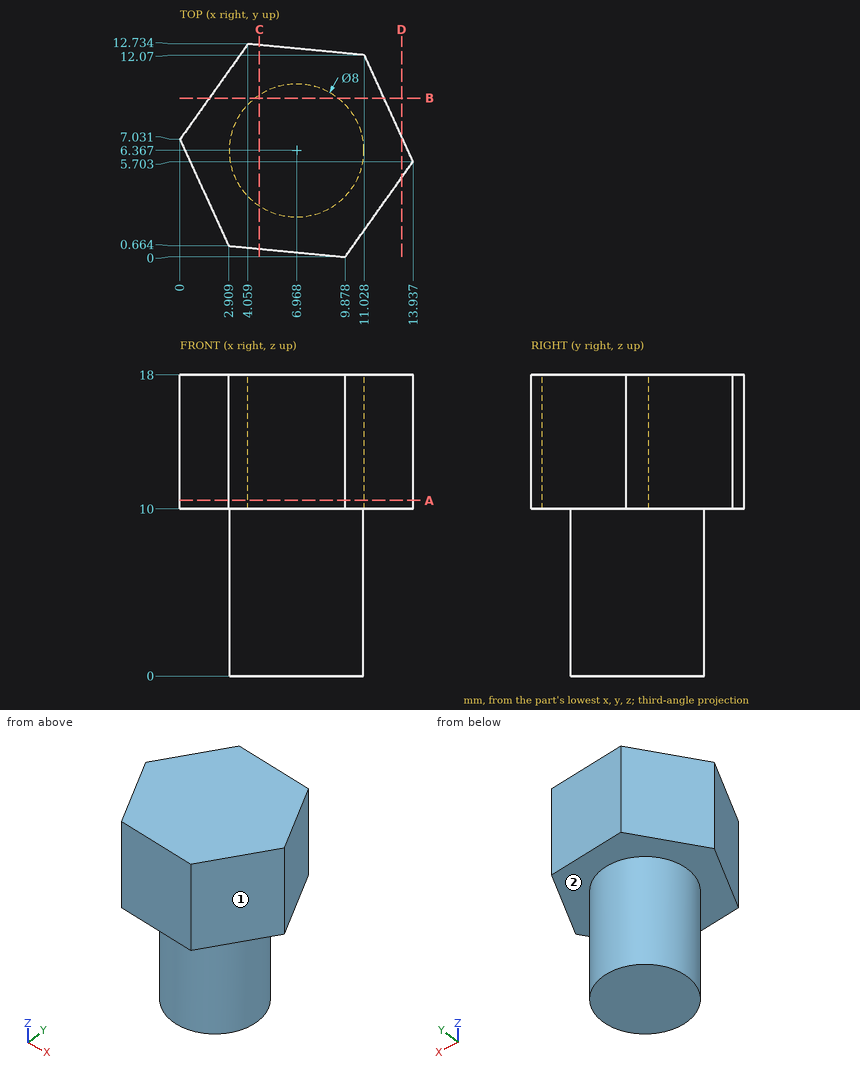
Can you work these out from the drawing? Everything is in mm from the part's minimum corner. A direction names the side the tool comes from. Round coordinates to 2 decimals unless told otherwise and drop trailing zeros. Order: outer loops, then holes, each group sorted by start corner. A loop starts at its lowest first (then second) coordinate and runs counter-clockwise, first axis right, second up. Notation, with made-up numbers: (-15.75, 24.25) -> (32.25, 24.25) arc R27 cw to (32.25, 49.25) -> close; hole circle Ø11 at (-1.75, 9.5). An arc over 180 degrees is marked (long way). Return JSON: item names as keys, results as strings. Group by question number.
1. If we section it at C-C, the plane x = 4.75: Write out the boundary of the cut face in (y, z) (1 decimal).
2. If we section it at A-A, the plane z = 10.5: Write out the boundary of the cut face in (x, y).
3. If we section it at D-D, the plane x = 13.25: Write out the boundary of the cut face in (y, z).
4. Which directions (+Z, -Z, +X, -X, +Y, -Y) give clear straight access to the entire face, cutting with the end or side of a thin tool? Please do the marked faces 1 and 2.
5. If we section it at B-B, the plane y = 9.5: Write out the boundary of the cut face in (x, z) (1 decimal), then the cut area to 3 significant figures.
6. I need wall thicknesses on line 1 (Z direction, x = 1.25, y = 4.75); line 2 (X direction, y = 11.5, z = 16); line 3 (X direction, y = 5, z = 3.25). Which ranges of each line are inside material? Lowest first, please. Write a range as [from, to].
7. Will these pins go through, and if not, where does the flat tip stop? pin 1 (4 mm diameter, centred on x = 7, z = 13, fed in from +Y); pin 2 (1 mm diameter, centred on x = 3.5, z = 15, fed in from +Y); pin 3 (3 mm diameter, centred on x = 11.5, z = 8, fed in from -Y) (1 decimal).
Output values:
{
 "1": {"outline": "(0.5, 10) -> (3, 10) -> (3, 0) -> (9.7, 0) -> (9.7, 10) -> (12.7, 10) -> (12.7, 18) -> (0.5, 18) -> close"},
 "2": {"outline": "(0, 7.03) -> (2.91, 0.66) -> (9.88, 0) -> (13.94, 5.7) -> (11.03, 12.07) -> (4.06, 12.73) -> close"},
 "3": {"outline": "(4.74, 10) -> (7.21, 10) -> (7.21, 18) -> (4.74, 18) -> close"},
 "4": {"face 1": "+Z, -Z, +X, -Y", "face 2": "-Z"},
 "5": {"outline": "(1.8, 10) -> (4.5, 10) -> (4.5, 0) -> (9.5, 0) -> (9.5, 10) -> (12.2, 10) -> (12.2, 18) -> (1.8, 18) -> close", "area": "133 mm²"},
 "6": {"line 1": "[10, 18]", "line 2": "[3.18, 11.29]", "line 3": "[3.21, 10.73]"},
 "7": {"pin 1": "y = 12.64", "pin 2": "y = 12.65", "pin 3": "y = 3.8"}
}
